Here's how the part is built. I have some questions about the finished solid (model axes, mm). A direction names the side the tool comes from. Give positions to 0.01 mm unless a question says otherwise; leave off trailing zeros. Loops run counter-clockwise (first coordinate to the right, second up) from the corner with the lowest first, then second, coordinate; pieces in that order, holes last. Notation, with made-up numbers: (29, -33.5) -> (38, -33.5) arc R19 ccw to (38, -14.5) -> close; hole circle Ø4 at (16, 15.25). An arc over 180 degrees is marked (long way). Answer in a Markdown table with one row per item. Add a question column.
Item 1: If I drill on line 1 (X direction, y = 0, z = 14.25); line 2 (Z direction, x = -5.25, y = 2.25); line 3 (Y direction, x = 8.25, z = 7.75), over which ranges is the centre line in solid material (lowest first)?
Item 2: For P1, Ø6, axis at x = -4.5, z = 11.5, coming from the -Y side; P2, Ø1.5, axis at x = 7.5, y = 1, coming from the -Z side; P3, Ø4, axis at x = 7.5, z = 13, coming from the -Y side; P4, Ø4, axis at x = -1, z = 4.5, coming from the +Y side, each with a flat end and sliding along its axis, tell me the tip position at first contact or that it passes through.
Item 3: If we section it at D-D (z = 9.25): Write out the boundary of the cut face in (x, y), then the cut area to 3 significant figures.
Item 4: If we section it at B-B (y = 0): Write out the boundary of the cut face in (x, z), then the cut area to 3 significant figures.
Item 5: Which directions (+Z, -Z, +X, -X, +Y, -Y) give clear straight access to the entire face, cutting with the end or side of a thin tool? Please do faces 4 (the face through (6, 2.5, 10)), 5 (the face through (-6, -2.5, 10)), 6 (the face through (-0.596, -2.685, 12.465)).
Item 6: If we section it at C-C (z = 10.75): Write out the boundary of the cut face in (x, y), then the cut area to 3 significant figures.
Item 7: We'd pull the mould along X, two halves only. Please class faces 1 (the face through (-10, 0, 10)), 2 (the face through (7, 0, 5)), 3 (the face through (2.003, 0.631, 5.184)): released by +X, released by -X, zero draft, split by the parting line, or undercut.
Item 8: If we section it at A-A (x = 0): Write out the boundary of the cut face in (y, z), then the cut area to 3 significant figures.
```python
from build123d import *

# Parameters (mm, degrees)
F0_R     = 5
F0_R_2   = 2.1
F1_DEPTH = 10
F2_R     = 2.75
F3_DEPTH = 5
F4_SIZE  = 0.5


with BuildPart() as f1:
    # F0 (on Top) → F1 (new body)
    with BuildSketch(Plane.XY):
        Circle(F0_R)
        Circle(F0_R_2, mode=Mode.SUBTRACT)
    extrude(amount=F1_DEPTH)

    # F2 (on face) → F3 (join, symmetric)
    with BuildSketch(Plane.XY.offset(10)):
        with BuildLine():
            ThreePointArc((5, 0), (4.829629, 1.294095), (4.330127, 2.5))
            ThreePointArc((4.330127, 2.5), (0, 5), (-4.330127, 2.5))
            ThreePointArc((-4.330127, 2.5), (-5, 0), (-4.330127, -2.5))
            ThreePointArc((-4.330127, -2.5), (0, -5), (4.330127, -2.5))
            ThreePointArc((4.330127, -2.5), (4.829629, -1.294095), (5, 0))
        make_face()
        Circle(F2_R, mode=Mode.SUBTRACT)
        with BuildLine():
            Line((8.5, 2.5), (4.330127, 2.5))
            ThreePointArc((4.330127, 2.5), (4.829629, 1.294095), (5, 0))
            ThreePointArc((5, 0), (4.829629, -1.294095), (4.330127, -2.5))
            Line((4.330127, -2.5), (8.5, -2.5))
            ThreePointArc((8.5, -2.5), (9.56066, -2.06066), (10, -1))
            Line((10, -1), (10, 1))
            ThreePointArc((10, 1), (9.56066, 2.06066), (8.5, 2.5))
        make_face()
        with BuildLine():
            ThreePointArc((-4.330127, -2.5), (-5, 0), (-4.330127, 2.5))
            Line((-4.330127, 2.5), (-8.5, 2.5))
            ThreePointArc((-8.5, 2.5), (-9.56066, 2.06066), (-10, 1))
            Line((-10, 1), (-10, -1))
            ThreePointArc((-10, -1), (-9.56066, -2.06066), (-8.5, -2.5))
            Line((-8.5, -2.5), (-4.330127, -2.5))
        make_face()
    extrude(amount=F3_DEPTH, both=True)

    # F4
    f4_edges = [f1.edges().sort_by_distance(p)[0] for p in [
        (-5, 0, 0),
        (-2.1, 0, 0),
    ]]
    chamfer(f4_edges, length=F4_SIZE)


solid = f1.part
```
Recorded:
| question | item | result |
|---|---|---|
| 1 | line 1 | x = -10 to -2.75, 2.75 to 10 |
| 1 | line 2 | z = 5 to 15 |
| 1 | line 3 | y = -2.5 to 2.5 |
| 2 | P1 | stops at y = -4.77 |
| 2 | P2 | stops at z = 5 |
| 2 | P3 | stops at y = -2.5 |
| 2 | P4 | stops at y = 5 |
| 3 | outline | (-10, -1) arc R1.5 ccw to (-8.5, -2.5) -> (-4.33, -2.5) arc R5 ccw to (4.33, -2.5) -> (8.5, -2.5) arc R1.5 ccw to (10, -1) -> (10, 1) arc R1.5 ccw to (8.5, 2.5) -> (4.33, 2.5) arc R5 ccw to (-4.33, 2.5) -> (-8.5, 2.5) arc R1.5 ccw to (-10, 1) -> close; hole circle Ø4.2 at (0, 0) |
| 3 | area | 115 mm^2 |
| 4 | outline | (-10, 5) -> (-5, 5) -> (-5, 0.5) -> (-4.5, 0) -> (-2.6, 0) -> (-2.1, 0.5) -> (-2.1, 10) -> (-2.75, 10) -> (-2.75, 15) -> (-10, 15) -> close; (2.1, 0.5) -> (2.6, 0) -> (4.5, 0) -> (5, 0.5) -> (5, 5) -> (10, 5) -> (10, 15) -> (2.75, 15) -> (2.75, 10) -> (2.1, 10) -> close |
| 4 | area | 180 mm^2 |
| 5 | face 4 | +Z, -Z, +X, +Y |
| 5 | face 5 | +Z, -Z, -X, -Y |
| 5 | face 6 | +Z |
| 6 | outline | (-10, -1) arc R1.5 ccw to (-8.5, -2.5) -> (-4.33, -2.5) arc R5 ccw to (4.33, -2.5) -> (8.5, -2.5) arc R1.5 ccw to (10, -1) -> (10, 1) arc R1.5 ccw to (8.5, 2.5) -> (4.33, 2.5) arc R5 ccw to (-4.33, 2.5) -> (-8.5, 2.5) arc R1.5 ccw to (-10, 1) -> close; hole circle Ø5.5 at (0, 0) |
| 6 | area | 105 mm^2 |
| 7 | face 1 | released by -X |
| 7 | face 2 | zero draft |
| 7 | face 3 | undercut |
| 8 | outline | (-5, 0.5) -> (-4.5, 0) -> (-2.6, 0) -> (-2.1, 0.5) -> (-2.1, 10) -> (-2.75, 10) -> (-2.75, 15) -> (-5, 15) -> close; (2.1, 0.5) -> (2.6, 0) -> (4.5, 0) -> (5, 0.5) -> (5, 15) -> (2.75, 15) -> (2.75, 10) -> (2.1, 10) -> close |
| 8 | area | 80.0 mm^2 |
